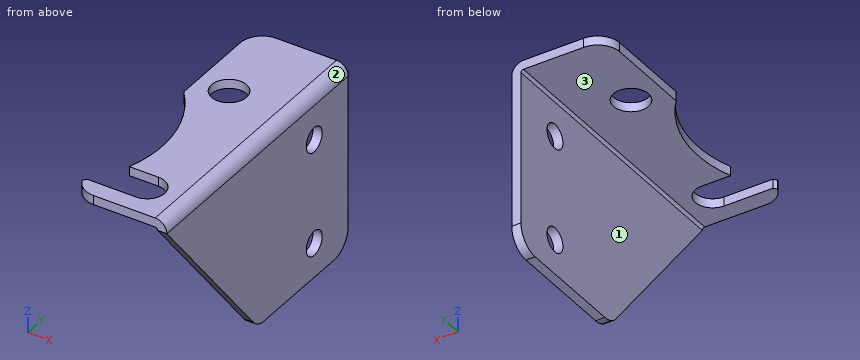
```python
from build123d import *

# Parameters (mm, degrees)
SKETCH2_R          = 5.08
BASE_FLANGE2_DEPTH = 2.65684
EDGE_FLANGE2_DEPTH = 81.28
SKETCH18_R         = 3.556
CUT_EXTRUDE1_DEPTH = 2.65684
FILLET1_R          = 6.35


# Sheet-metal steps are written as plain solids
with BuildPart() as part:
    # Sketch2 → Base-Flange2 (new body)
    with BuildSketch(Plane.XY):
        with BuildLine():
            Line((-11.8872, -36.520431679), (-11.8872, -40.64))
            Line((-11.8872, -40.64), (11.8872, -40.64))
            Line((11.8872, -40.64), (11.8872, 40.64))
            Line((11.8872, 40.64), (-11.8872, 40.64))
            Line((-11.8872, 40.64), (-11.8872, 8.936031679))
            ThreePointArc((-11.8872, 8.936031679), (-4.075086446, -7.37142183), (-5.465240134, -25.4))
            Line((-5.465240134, -25.4), (2.9972, -25.4))
            ThreePointArc((2.9972, -25.4), (8.0772, -30.48), (2.9972, -35.56))
            Line((2.9972, -35.56), (-11.093291287, -35.56))
            ThreePointArc((-11.093291287, -35.56), (-11.485961922, -36.043756834), (-11.8872, -36.520431679))
        make_face()
        with Locations((-2.8448, 15.24)):
            Circle(SKETCH2_R, mode=Mode.SUBTRACT)
    extrude(amount=-BASE_FLANGE2_DEPTH)

    # Edge-Flange2 section (across the edge) → Edge-Flange2 (add)
    with BuildSketch(Plane(origin=(12.6238, 40.64, -2.65684), x_dir=(-1, 0, 0), z_dir=(0, -1, 0))):
        with BuildLine():
            Line((-2.65684, 0.7366), (-2.65684, 51.31816))
            Line((-2.65684, 51.31816), (0, 51.31816))
            Line((0, 51.31816), (0, 0.7366))
            ThreePointArc((0, 0.7366), (0.215745145, 0.215745145), (0.7366, 0))
            Line((0.7366, 0), (0.7366, -2.65684))
            ThreePointArc((0.7366, -2.65684), (-1.662924436, -1.662924436), (-2.65684, 0.7366))
        make_face()
    extrude(amount=EDGE_FLANGE2_DEPTH)

    # Sketch18 → Cut-Extrude1 (cut)
    with BuildSketch(Plane(origin=(15.28064, 0, 0), x_dir=(0, 0, -1), z_dir=(1, 0, 0))):
        with Locations((13.44422, 25.4)):
            Circle(SKETCH18_R)
        with Locations((43.92422, 25.4)):
            Circle(SKETCH18_R)
        Polygon((53.975, 0), (53.975, -40.64), (3.39344, -40.64), align=None)
    extrude(amount=-CUT_EXTRUDE1_DEPTH, mode=Mode.SUBTRACT)

    # Fillet1
    # the kernel refuses this fillet: 6.35 mm, written as the material it takes off along each edge
    with BuildSketch(Plane(origin=(-11.8872, 40.64, 15.875), x_dir=(0, -1, 0), z_dir=(0, 0, -1)), Plane(origin=(31.15564, 40.64, -53.975), x_dir=(0, 0, 1), z_dir=(-1, 0, 0))) as fillet1_piece_1:
        with BuildLine():
            CenterArc((FILLET1_R, -FILLET1_R), FILLET1_R, 90, 90)
            Line((0, -FILLET1_R), (-FILLET1_R * 0.02, -FILLET1_R))
            Line((-FILLET1_R * 0.02, -FILLET1_R), (-FILLET1_R * 0.02, FILLET1_R * 0.02))
            Line((-FILLET1_R * 0.02, FILLET1_R * 0.02), (FILLET1_R, FILLET1_R * 0.02))
            Line((FILLET1_R, FILLET1_R * 0.02), (FILLET1_R, 0))
        make_face()
    extrude(amount=34.40684, mode=Mode.SUBTRACT)
    with BuildSketch(Plane(origin=(-11.8872, -40.64, 14.863477581), x_dir=(0, 1, 0), z_dir=(0, 0, -1))) as fillet1_piece_2:
        with BuildLine():
            CenterArc((6.35, 5.945391032), FILLET1_R, 180, 69.436266332)
            Line((0, 5.945391032), (-0.127, 5.945391032))
            Line((-0.127, 5.945391032), (-0.127, 0))
            Line((-0.127, 0), (0, -0.127))
            ThreePointArc((0, -0.127), (2.059784161, -0.127), (4.074959688, -0.118907821))
            Line((4.074959688, -0.118907821), (4.119568321, 0))
        make_face()
    extrude(amount=32.383795161, mode=Mode.SUBTRACT)
    with BuildSketch(Plane(origin=(22.890020574, 0, -53.975), x_dir=(-2.7142023433715092e-15, -0.6263358882152561, 0.7795533048699147), z_dir=(-1, 0, 0))) as fillet1_piece_3:
        with BuildLine():
            CenterArc((FILLET1_R * 0.479331059788, FILLET1_R), FILLET1_R, 218.780305406, 51.219694594)
            Line((-FILLET1_R * 0.300222245082, FILLET1_R * 0.373664111785), (-FILLET1_R * 0.315813311179, FILLET1_R * 0.36113739402))
            Line((-FILLET1_R * 0.315813311179, FILLET1_R * 0.36113739402), (-FILLET1_R * 0.00958662119577, -FILLET1_R * 0.02))
            Line((-FILLET1_R * 0.00958662119577, -FILLET1_R * 0.02), (FILLET1_R * 0.479331059788, -FILLET1_R * 0.02))
            Line((FILLET1_R * 0.479331059788, -FILLET1_R * 0.02), (FILLET1_R * 0.479331059788, 0))
        make_face()
    extrude(amount=17.875601148, mode=Mode.SUBTRACT)


solid = part.part
```
Verification items for the finished model (mm, model axes). Face numbers are marked on the shaded views. Give positions to 0.01 mm unless a question says otherwise; leave off trailing zeros. Order: outer loops, then holes, each group sorted by start corner. A loop starts at its lowest first (then second) coordinate and runs counter-clockwise, first axis right, second up. Notation, with made-up numbers: (-26, 33) -> (13, 33) arc R21 cw to (13, 47) -> close; hole circle Ø1 at (30, 45.25). An arc over 180 degrees is marked (long way). Use a Markdown table: item, result.
1) Mould release check, pull along Z, two halves, no side actions. Record for the marked faces 1, 2 and 3: pulls with the +Z half, pulls with the -Z half, needs draft (parallel to the pull), parting line crosses it, or undercut.
Results:
| item | result |
|---|---|
| face 1 | needs draft |
| face 2 | pulls with the +Z half |
| face 3 | pulls with the -Z half |
2) Section check D-D, the plane x = -4.5. Record the boundary of the cut face in (y, z), then the cut area to 3 significant figures.
Results:
| item | result |
|---|---|
| outline | (-40.64, -2.66) -> (-35.56, -2.66) -> (-35.56, 0) -> (-40.64, 0) -> close; (-25.4, -2.66) -> (-22.17, -2.66) -> (-22.17, 0) -> (-25.4, 0) -> close; (-5.41, -2.66) -> (10.44, -2.66) -> (10.44, 0) -> (-5.41, 0) -> close; (20.04, -2.66) -> (40.64, -2.66) -> (40.64, 0) -> (20.04, 0) -> close |
| area | 119 mm² |
3) Material ranges on probe 1 along X at (y, z) = (14, -47); probe 2 along Z at (x, y) = (10.75, -28.5); probe 3 along Y at (x, z) = (14.25, -15), recorded low to high.
Results:
| item | result |
|---|---|
| probe 1 | 12.62 to 15.28 |
| probe 2 | -2.66 to 0 |
| probe 3 | -31.31 to 22.2, 28.6 to 40.64 |
4) Section check A-A, the plane y = 15.24. Record the boundary of the cut face in (x, z) (3 decimals).
Results:
| item | result |
|---|---|
| outline | (-11.887, -2.657) -> (-7.925, -2.657) -> (-7.925, 0) -> (-11.887, 0) -> close; (2.235, -2.657) -> (11.887, -2.657) arc R0.737 cw to (12.624, -3.393) -> (12.624, -53.975) -> (15.281, -53.975) -> (15.281, -3.393) arc R3.393 ccw to (11.887, 0) -> (2.235, 0) -> close |
5) Section check C-C, the plane z = -44.5. Record the boundary of the cut face in (x, y).
Results:
| item | result |
|---|---|
| outline | (12.62, -7.61) -> (15.28, -7.61) -> (15.28, 21.89) -> (12.62, 21.89) -> close; (12.62, 28.91) -> (15.28, 28.91) -> (15.28, 40.64) -> (12.62, 40.64) -> close |
6) Depth check by flat-ended pin: pin 1 Ø8 at (y, z) = (25.4, -43.92) entering from -X; pin 2 Ø4 at (x, y) = (-2.5, -11.5) entering from -Z. Enter the tip coordinate at first touch or a pass-through.
Results:
| item | result |
|---|---|
| pin 1 | x = 12.62 |
| pin 2 | z = -2.66 |
7) Section check B-B, the plane x = -9.75. Record the boundary of the cut face in (y, z).
Results:
| item | result |
|---|---|
| outline | (-39.37, -2.66) -> (-35.56, -2.66) -> (-35.56, 0) -> (-39.37, 0) -> close; (6.17, -2.66) -> (39.04, -2.66) -> (39.04, 0) -> (6.17, 0) -> close |
